Autodesk Inventor part; units mm, degrees
ref_plane "Work Plane1" through (30.1625, 0, 0) normal (0, 0, -1) x (1, 0, 0)
ref_plane "YZ Plane" through (0, 0, 0) normal (1, 0, 0) x (0, 1, 0)
ref_plane "XZ Plane" through (0, 0, 0) normal (0, 1, 0) x (-1, 0, 0)
sketch "Schizzo1" plane through (0, 0, 0) normal (0, 0, 1) x (1, 0, 0)
  line L0 (-5, 0) -> (30, 0)
  line L1 (30, 0) -> (30, 4)
  line L2 (30, 4) -> (2.5, 4)
  line L3 (2.5, 4) -> (1.7331, 3.6618)
  line L4 (1.7331, 3.6618) -> (0, 3.6618)
  line L5 (0, 3.6618) -> (0, 6.5)
  line L6 (-12, 0) -> (37, 0)
  line L7 (0, -1.3) -> (0, 7.8)
  line L8 (-5, 0) -> (-5, 6.0626)
  line L9 (0, 6.5) -> (-5, 6.0626)
  line L10 (2.5, 4) -> (0, 4) construction
  dimension "d0" = 30
  dimension "d1" = 27.5
  dimension "d2" = 0.7669
  dimension "d3" = 5
  dimension "d4" = 8
  dimension "d5" = 7.3235
  dimension "d9" = 13
  dimension "d10" = 5
revolve "Corpo" add sketch "Schizzo1" angle 360 about axis through (-5, 0, 0) along (1, 0, 0)
sketch "Schizzo2" plane through (-5, 0, 0) normal (-1, 0, 0) x (0, 0, 1)
  circle A0 centre (0, 0) radius 6.5
  line L0 (0, 0) -> (0, 6.0626)
  line L1 (-6.5, 1) -> (6.5, 1)
  line L2 (6.5, 1) -> (6.5, -1)
  line L3 (6.5, -1) -> (-6.5, -1)
  line L4 (-6.5, -1) -> (-6.5, 1)
  line L5 (-6.5, 0) -> (6.5, 0) construction
  line L6 (0, 1) -> (0, -1) construction
  dimension "d11" = 2
  dimension "d12" = 13
fillet "Raccordo1" radius 0.4 1 edges at (-5, -6.0626, 0)
extrude "Intaglio" cut sketch "Schizzo2" against normal blind 2 contours A0 L3 L1 | L2 L3 A0 | A0 L1 L2 | A0 L4 L1 | L3 L4 A0
thread "Filettatura"
chamfer "Smusso1" distance 3.95 distance2 0.7669 1 edges at (30, -4, 0) measured on face at (30, 0.998, 0.8842)
ref_plane "Work Plane1" through (30.1625, 0, 0) normal (0, 0, -1) x (1, 0, 0)
equation "\"d11\" = SBR"
equation "\"d12\" = KOD"
equation "\"d14\" = RR"
equation "\"d19\" = STI"
equation "\"d15\" = GEL"
equation "\"d17\" = -0.5 * SPD + 0.5 * GD"
equation "\"d0\" = NLG"
equation "\"d1\" = GEL"
equation "\"d3\" = KOH"
equation "\"d4\" = GD"
equation "\"d5\" = BDM"
equation "\"d9\" = KOD"
equation "\"d10\" = KEWI"
equation "\"GD\" = NND"
equation "\"NLG\" = 30"
equation "\"GEL\" = 27.5"
equation "\"KOD\" = 13"
equation "\"KOH\" = 5"
equation "\"GAL\" = 0.61345 * PTC"
equation "\"SPD\" = 0.1"
equation "\"BDM\" = 7.3235"
equation "\"GUL\" = 0.61345 * PTC"
equation "\"RR\" = 0.4"
equation "\"SBR\" = 2"
equation "\"STI\" = 2"
equation "\"KEWI\" = 5deg"
equation "\"THREADDIA\" = 8"
equation "\"TOA\" = 30deg"
equation "\"PTC\" = 1.25"
equation "\"NND\" = 8"
equation "\"GD1\" = THREADDIA - 1.2269 * PTC"
properties part number "IS 1366 - M8 x 30" material "Acciaio, Dolce"
Can you work these out from the model? Positions are in its coordinate system, mm. A direction names the side the tool comes from. Coordinates: 2 decimals unless noted, no trailing zeros. Loops run counter-clockwise (first coordinate to the right, second up) from the corner with the lowest first, then second, coordinate; pieces in that order, holes last. Notation, with made-up numbers: (-23, 81.25) - (22, 81.25) arc R26 cw to (22, 114.25) - close; hole circle Ø7 at (5, 26.25). An arc over 180 degrees is marked (long way). Put each result on its own line as item: value. Start each with the question number.
Item 1: If we mould it in two halves opening along Y, with no side actions, what happens to faces 4 (the face through (-4, 1, 0)), 5 (the face through (-4, -1, 0)), 6 (the face through (15.679, -0.867, 3.905)), 7 (the face through (-5, -3, 0))? For each: +Y half, -Y half, draft (parallel to the pull), parting line (faces both ways), or undercut.
Item 2: For pin 1 (4 mm diameter, centred on y = 1, z = -2.5, fed in from +X); pin 2 (6 mm diameter, centred on x = -0.5, y = -3.5, fed in from -Z); pin 3 (1.5 mm diameter, centred on x = 15, z = 2.5, fed in from -Y), each with a flat end and sliding along its axis, tell me the tip position at first contact or that it passes through.
Item 3: Which directions (+Z, -Z, +X, -X, +Y, -Y) give clear straight access to the entire face, cutting with the end or side of a thin tool? Please do faces 1 (the face through (0.854, 3.493, -1.1)), 2 (the face through (-3, 0, 0)), 3 (the face through (-5, 3, 0)).
Item 4: If I drill on line 1 along X through (y, z) = (3.5, -2); line 2 along X through (y, z) = (1.75, 3); line 3 along Y through (x, z) = (23.5, -0.25), over which ranges is the centre line in solid material (lowest first)?
Item 5: Suppose I cut it at A-A (x = 14.5). Please give me the cut outline in (y, z).
Here are the results:
1. face 4: undercut
1. face 5: undercut
1. face 6: parting line
1. face 7: draft
2. pin 1: x = 29.88
2. pin 2: z = -6.48
2. pin 3: y = -3.6
3. face 1: none
3. face 2: +Z, -Z, -X
3. face 3: +Z, -Z, -X, +Y, -Y
4. line 1: -5 to 0
4. line 2: -5 to 29.34
4. line 3: -3.99 to 3.99
5. outline: circle Ø8 at (0, 0)
